Check sheet for the modelled part. Datum: model origin and axes. Units: mm. Face numbers are marked on the shaded views. A direction names the side the tool comes from. Give positions to 0.01 mm unless a question says otherwise; leave off trailing zeros. Order: outer loops, then holes, each group sorted by start corner. A loop starts at its lowest first (then second) coordinate and runs counter-clockwise, first axis right, second up.
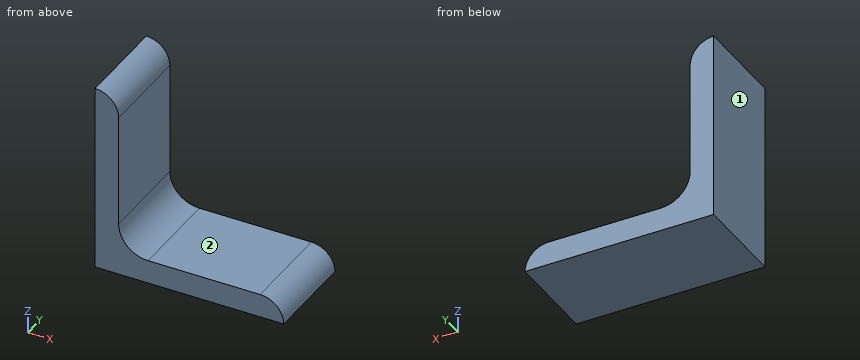
```python
from build123d import *

# Parameters (mm, degrees)
F1_DEPTH = 12.7
F2_R     = 6.34999
F3_R     = 7.9375


# Not quite as in the source:
# - a fillet or chamfer is up to 0.001 mm smaller than in the source, because OpenCascade refuses the exact size


with BuildPart() as f1:
    # F0 (on Front) → F1 (new body, symmetric)
    with BuildSketch(Plane.XZ):
        Polygon((6.35, 50.8), (0, 50.8), (0, 0), (50.8, 0), (50.8, 6.35), (6.35, 6.35), align=None)
    extrude(amount=F1_DEPTH, both=True)

    # F2 (radius 6.35 in the source; OpenCascade refuses exactly that, so slightly less here)
    f2_edges = [f1.edges().sort_by_distance(p)[0] for p in [
        (6.35, 0, 50.8),
        (50.8, 0, 6.35),
    ]]
    fillet(f2_edges, radius=F2_R)

    # F3
    f3_edges = [f1.edges().sort_by_distance(p)[0] for p in [
        (6.35, 0, 6.35),
    ]]
    fillet(f3_edges, radius=F3_R)


solid = f1.part
```
(1) Set-up check for the marked faces 1 and 2: record each of +Z, -Z, +X, -X, +Y, -Y from which the full face is reachable in a straight line by a thin tool's end or side.
Response values:
face 1: +Z, -Z, -X, +Y, -Y
face 2: +Z, +X, +Y, -Y
(2) Cross-section at C-C on z = 46.5. Enter the section's corners in (x, y).
Response values:
outline: (0, -12.7) - (6.01, -12.7) - (6.01, 12.7) - (0, 12.7) - close
(3) Gauge pin test, flat ends, axial feed: pin 1 Ø8 at (y, z) = (3, 30.5) entering from -X; pin 2 Ø1 at (x, y) = (35, -6.5) entering from +Z; pin 3 Ø1 at (x, z) = (13.5, 7.5) entering from -Y. Record the tip position at first contact, or that the pin passes through.
Response values:
pin 1: stops at x = 0
pin 2: stops at z = 6.35
pin 3: passes through
(4) Cross-section at B-B on x = 23.5. Enter the section's corners in (y, z).
Response values:
outline: (-12.7, 0) - (12.7, 0) - (12.7, 6.35) - (-12.7, 6.35) - close
(5) Material ranges on L1, parallel to X at y = -9, z = 41.5, recorded low to high.
Response values:
L1: x = 0 to 6.35
